Here's how the part is built. I have some questions about the finished solid (model axes, mm). Face numbers are marked on the shaded views. A direction names the side the tool comes from. Round coordinates to 2 decimals unless told otherwise and drop trailing zeros. Order: outer loops, then holes, each group sorted by start corner. A loop starts at its lowest first (then second) coordinate and runs counter-clockwise, first axis right, second up. Notation, with made-up numbers: (-40, 56.25) -> (13, 56.25) arc R19 cw to (13, 77.25) -> close; hole circle Ø11 at (44, 40.5). An arc over 180 degrees is marked (long way). Use a Markdown table: item, result. Add a question column.
from build123d import *

# Parameters (mm, degrees)
SKETCH_W        = 20
SKETCH_H        = 15
PAD_DEPTH       = 2
SKETCH001_W     = 20
SKETCH001_H     = 2
PAD001_DEPTH    = 12
POCKET002_DEPTH = 5
COPYSKETCH005_R = 2
POCKET_DEPTH    = 5
FILLET_R        = 1
FILLET001_R     = 1
FILLET002_R     = 1
FILLET003_R     = 1


with BuildPart() as part:
    # Sketch → Pad (new body)
    with BuildSketch(Plane.XY):
        Rectangle(SKETCH_W, SKETCH_H)
    extrude(amount=PAD_DEPTH)

    # Sketch001 (on Face6 of Pad) → Pad001 (join)
    with BuildSketch(Plane.XY.offset(2)):
        with Locations((0, -6.5)):
            Rectangle(SKETCH001_W, SKETCH001_H)
    extrude(amount=PAD001_DEPTH)

    # Sketch004 → Pocket002 (cut)
    with BuildSketch(Plane(origin=(0, -2.5, 0), x_dir=(-1, 0, 0), z_dir=(0, 1, 0))):
        with BuildLine():
            Line((-6, 6.828421), (6, 6.828421))
            ThreePointArc((6, 6.828421), (8, 8.828421), (6, 10.828421))
            Line((6, 10.828421), (-6, 10.828421))
            ThreePointArc((-6, 10.828421), (-8, 8.828421), (-6, 6.828421))
        make_face()
    extrude(amount=-POCKET002_DEPTH, mode=Mode.SUBTRACT)

    # CopySketch005 → Pocket (cut)
    with BuildSketch(Plane.XY.offset(2)):
        with Locations((0, 2.587535)):
            Circle(COPYSKETCH005_R)
    extrude(amount=-POCKET_DEPTH, mode=Mode.SUBTRACT)

    # Fillet
    fillet_edges = [part.edges().sort_by_distance(p)[0] for p in [
        (-10, 7.5, 1),
    ]]
    fillet(fillet_edges, radius=FILLET_R)

    # Fillet001
    fillet001_edges = [part.edges().sort_by_distance(p)[0] for p in [
        (10, 7.5, 1),
    ]]
    fillet(fillet001_edges, radius=FILLET001_R)

    # Fillet002
    fillet002_edges = [part.edges().sort_by_distance(p)[0] for p in [
        (-10, -6.5, 14),
    ]]
    fillet(fillet002_edges, radius=FILLET002_R)

    # Fillet003
    fillet003_edges = [part.edges().sort_by_distance(p)[0] for p in [
        (10, -6.5, 14),
    ]]
    fillet(fillet003_edges, radius=FILLET003_R)


solid = part.part
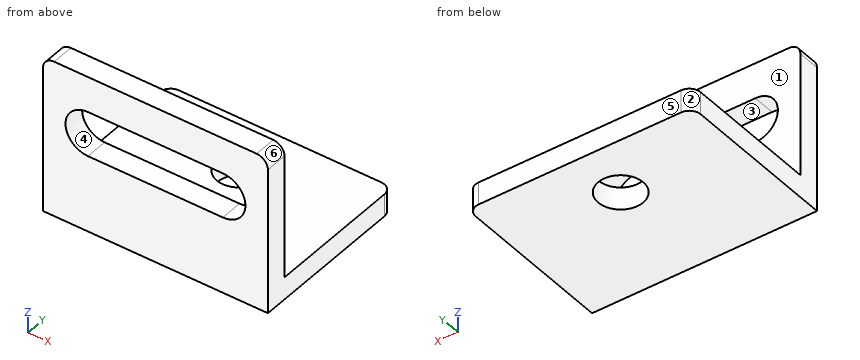
(1) I want a section at C-C on x = -5.5. List the corners of the cut face in (y, z) for me, and give its area (3 significant figures).
(2) If we mould it in two halves opening along Z, with no side actions, what happens to the marked faces 4, 5 and 6? For each: pulls with the +Z half, pulls with the -Z half, needs draft (parallel to the pull), parting line crosses it, or undercut.
(3) On a 3-axis mill with a long thin cutter (end or side, diameter ignored), from which of +Z, -Z, +X, -X, +Y, -Y can I reach the whole of each face in a straight line? I mean the marked faces 1, 2 and 3. Say none if no direction works.
(4) I'm going to push flat-ended pins straight in: P1, Ø4.5, axis at x = 0, y = 2.59, coming from the +Z side; P2, Ø2, axis at x = -6.5, z = 5, coming from the +Y side; P3, Ø1.5, axis at y = -4.5, z = 6.5, coming from the +X side. Where does each tip first touch, or does it pass through?
(5) I want a section at D-D on z = 10.5. List the corners of the cut face in (x, y) for me, and give its area (3 significant figures).
(6) I want a section at B-B on y = 3.75. List the corners of the cut face in (x, z) for me, and give its area (3 significant figures).
(7) I want a section at A-A on x = 0. List the corners of the cut face in (y, z) for me, and give its area (3 significant figures).
(8) Please list where these lines run through material, in increasing order: probe 1 along Y at (x, z) = (0, 0.65); probe 2 along Z at (x, y) = (3.25, -6.25); probe 3 along Z at (x, y) = (2.25, -5.25). Write a range as from..to.
Output:
| question | item | result |
|---|---|---|
| 1 | outline | (-7.5, 0) -> (7.5, 0) -> (7.5, 2) -> (-5.5, 2) -> (-5.5, 6.83) -> (-7.5, 6.83) -> close; (-7.5, 10.83) -> (-5.5, 10.83) -> (-5.5, 14) -> (-7.5, 14) -> close |
| 1 | area | 46.0 mm² |
| 2 | face 4 | undercut |
| 2 | face 5 | needs draft |
| 2 | face 6 | pulls with the +Z half |
| 3 | face 1 | +Z, +X, -X, +Y |
| 3 | face 2 | +Z, -Z, -X, +Y |
| 3 | face 3 | +Y, -Y |
| 4 | P1 | z = 2 |
| 4 | P2 | y = -5.5 |
| 4 | P3 | through |
| 5 | outline | (-10, -7.5) -> (-7.1, -7.5) -> (-7.1, -5.5) -> (-10, -5.5) -> close; (7.1, -7.5) -> (10, -7.5) -> (10, -5.5) -> (7.1, -5.5) -> close |
| 5 | area | 11.6 mm² |
| 6 | outline | (-10, 0) -> (-1.63, 0) -> (-1.63, 2) -> (-10, 2) -> close; (1.63, 0) -> (10, 0) -> (10, 2) -> (1.63, 2) -> close |
| 6 | area | 33.5 mm² |
| 7 | outline | (-7.5, 0) -> (0.59, 0) -> (0.59, 2) -> (-5.5, 2) -> (-5.5, 6.83) -> (-7.5, 6.83) -> close; (-7.5, 10.83) -> (-5.5, 10.83) -> (-5.5, 14) -> (-7.5, 14) -> close; (4.59, 0) -> (7.5, 0) -> (7.5, 2) -> (4.59, 2) -> close |
| 7 | area | 38.0 mm² |
| 8 | probe 1 | -7.5..0.59, 4.59..7.5 |
| 8 | probe 2 | 0..6.83, 10.83..14 |
| 8 | probe 3 | 0..2 |
